```python
from build123d import *

# Parameters (mm, degrees)
SKETCH018_R   = 4
SKETCH018_R_2 = 1.5
SKETCH018_R_3 = 12
PAD_DEPTH     = 10


with BuildPart() as part:
    # Sketch018 → Pad (new body)
    with BuildSketch(Plane(origin=(0, 0, 0), x_dir=(0, -1, 0), z_dir=(-1, 0, 0))):
        with BuildLine():
            ThreePointArc((19.148224, 17.588221), (0, 26), (-19.148224, 17.588221))
            ThreePointArc((-25.026104, 14.999977), (-21.816028, 15.678353), (-19.148224, 17.588221))
            ThreePointArc((-25.026104, 14.999977), (-40, 0), (-25.026104, -14.999977))
            ThreePointArc((-19.148224, -17.588221), (-21.816028, -15.678353), (-25.026104, -14.999977))
            ThreePointArc((-19.148224, -17.588221), (0, -26), (19.148224, -17.588221))
            ThreePointArc((25.026104, -14.999977), (21.816028, -15.678353), (19.148224, -17.588221))
            ThreePointArc((25.026104, -14.999977), (40, 0), (25.026104, 14.999977))
            ThreePointArc((19.148224, 17.588221), (21.816028, 15.678353), (25.026104, 14.999977))
        make_face()
        with Locations((-30, 0)):
            Circle(SKETCH018_R, mode=Mode.SUBTRACT)
        with Locations((30, 0)):
            Circle(SKETCH018_R, mode=Mode.SUBTRACT)
        with Locations((-15.5, 15.5)):
            Circle(SKETCH018_R_2, mode=Mode.SUBTRACT)
        with Locations((15.5, 15.5)):
            Circle(SKETCH018_R_2, mode=Mode.SUBTRACT)
        with Locations((-15.5, -15.5)):
            Circle(SKETCH018_R_2, mode=Mode.SUBTRACT)
        with Locations((15.5, -15.5)):
            Circle(SKETCH018_R_2, mode=Mode.SUBTRACT)
        Circle(SKETCH018_R_3, mode=Mode.SUBTRACT)
    extrude(amount=PAD_DEPTH)


solid = part.part
```
The listing builds one solid part. Answer for the finished solid, in the listing's coordinates (mm). Round coordinates to 2 decimals unless told otherwise and drop trailing zeros. Write each loop counter-clockwise with the first axis right and the second up, starting at its lowest first coordinate (ties: lowest second). Pieces come first, ordered by that corner, then holes. Notation, with made-up numbers: (-2, 51) -> (27, 51) arc R22 ccw to (27, 71) -> close; hole circle Ø1 at (78, -7). An arc over 180 degrees is marked (long way). Answer as a JSON object with one key per item and string values. Group by question number.
Q1. Section D-D (z = 8.5) is taken. Write down the section's boundary in (x, y).
Q2. Section C-C (x = -7) is taken. Write down the section's boundary in (y, z), plus the area to 3 significant figures.
Q3. Section A-A (z = 0) is taken. Write down the section's boundary in (x, y), plus the area to 3 significant figures.
Q4. Section B-B (y = 0) is taken. Write down the section's boundary in (x, z), plus the area to 3 significant figures.
Q5. Straight lines are drawn through the part: line 1 along Z through (x, y) = (-6.75, -0.5); line 2 along Y through (x, z) = (-3.5, -16.5); line 3 along Z through (x, y) = (-4.25, -15.5). For each, find the intervals that lie inside material, in ascending order.
Q6. Determine the mould class of faces 1 (the face through (-4.93, -21.86, -15.66)), 2 (the face through (-4.93, -14, -15.43)), 3 (the face through (-5, 40, 0)) for opening direction Z: pulls with the +Z half, pulls with the -Z half, needs draft (parallel to the pull), parting line crosses it, or undercut.
Check values:
{
 "1": {"outline": "(-10, -37.36) -> (0, -37.36) -> (0, -8.47) -> (-10, -8.47) -> close; (-10, 8.47) -> (0, 8.47) -> (0, 37.36) -> (-10, 37.36) -> close"},
 "2": {"outline": "(-25.03, -15) arc R8 cw to (-19.15, -17.59) arc R26 ccw to (19.15, -17.59) arc R8 cw to (25.03, -15) arc R15 ccw to (25.03, 15) arc R8 cw to (19.15, 17.59) arc R26 ccw to (-19.15, 17.59) arc R8 cw to (-25.03, 15) arc R15 ccw to start; hole circle Ø8 at (-30, 0); hole circle Ø3 at (-15.5, -15.5); hole circle Ø3 at (-15.5, 15.5); hole circle Ø24 at (0, 0); hole circle Ø3 at (15.5, -15.5); hole circle Ø3 at (15.5, 15.5); hole circle Ø8 at (30, 0)", "area": "2,290 mm^2"},
 "3": {"outline": "(-10, -40) -> (0, -40) -> (0, -34) -> (-10, -34) -> close; (-10, -26) -> (0, -26) -> (0, -12) -> (-10, -12) -> close; (-10, 12) -> (0, 12) -> (0, 26) -> (-10, 26) -> close; (-10, 34) -> (0, 34) -> (0, 40) -> (-10, 40) -> close", "area": "400 mm^2"},
 "4": {"outline": "(-10, -26) -> (0, -26) -> (0, -12) -> (-10, -12) -> close; (-10, 12) -> (0, 12) -> (0, 26) -> (-10, 26) -> close", "area": "280 mm^2"},
 "5": {"line 1": "-26 to -11.99, 11.99 to 26", "line 2": "-20.38 to -16.62, -14.38 to 14.38, 16.62 to 20.38", "line 3": "-20.87 to -17, -14 to 14, 17 to 20.87"},
 "6": {"face 1": "pulls with the -Z half", "face 2": "undercut", "face 3": "parting line crosses it"}
}
